Here's how the part is built. I have some questions about the finished solid (model axes, mm). Face numbers are marked on the shaded views. A direction names the side the tool comes from. Coordinates: 2 decimals unless noted, no trailing zeros. Order: outer loops, then holes, each group sorted by start corner. A loop starts at its lowest first (then second) coordinate and runs counter-clockwise, first axis right, second up. Notation, with made-up numbers: (64.5, 10) - (114.5, 10) arc R14 cw to (114.5, 25) - close; hole circle Ø10 at (4, -23). An arc over 180 degrees is marked (long way). Answer in a Markdown table with one row per item. Add a question column.
Item 1: I want a section at C-C (z = 4). Please give me the cut outline in (x, y) (3 decimals), plus the area to 3 significant figures.
Item 2: I want a section at D-D (z = 16). Please give me the cut outline in (x, y).
Item 3: On a 3-axis mill with a long thin cutter (end or side, diameter ignored), from which of +Z, -Z, +X, -X, +Y, -Y can I reach the whole of each face in a straight line? I mean the marked faces 4, 5, 6, 7 and 8. Say none if no direction works.
Item 4: If I drill on line 1 along Y through (x, z) = (54, 6); line 2 along Y through (x, z) = (22.5, 32); line 3 along Z through (x, y) = (24.5, -14.5), over which ranges is the centre line in solid material (lowest first)? Write a range as from..to.
Item 5: Will these pins go through, and if not, where does the flat tip stop? pin 1 Ø1 at (x, y) = (53, -6.5) entering from +Z; pin 2 Ø19 at (x, z) = (19, 27) entering from -Y; pin 3 Ø10 at (x, z) = (12.7, 31.75) entering from -Y; pin 4 Ø10 at (y, z) = (-7, 34.5) entering from +X.
Item 6: I want a section at A-A (y = -3). Please give me the cut outline in (x, z).
Item 7: Thinking about a two-plate mould opening in X: for the marked faces 1, 2 and 3, which applies, +X half, -X half, draft (parallel to the pull), parting line (faces both ways), or undercut?
Item 8: I want a section at B-B (z = 30). Please give me the cut outline in (x, y).
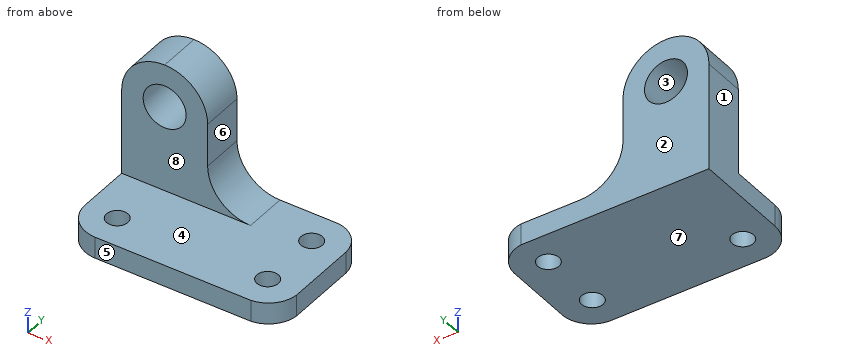
```python
from build123d import *

# Parameters (mm, degrees)
F0_W      = 63.5
F0_H      = 44.45
F1_DEPTH  = 38.1
F2_W      = 25.4
F2_H      = 38.1
F3_DEPTH  = 38.101
F5_W      = 25.4
F5_H      = 38.1
F6_DEPTH  = 38.101
F4_W      = 12.7
F4_H      = 25.4
F7_DEPTH  = 38.101
F8_R      = 6.35
F9_DEPTH  = 12.701
F10_R     = 3.175
F11_DEPTH = 6.351


# Not quite as in the source:
# - a feature names something its author has since deleted; it is built from what else it names


with BuildPart() as f1:
    # F0 (on Front) → F1 (new body)
    with BuildSketch(Plane.XZ):
        with Locations((31.75, 22.225)):
            Rectangle(F0_W, F0_H)
    extrude(amount=F1_DEPTH)

    # F2 (on face) → F3 (cut, through all)
    with BuildSketch(Plane.XZ.offset(38.1)):
        with Locations((50.8, 25.4)):
            Rectangle(F2_W, F2_H)
    extrude(amount=-F3_DEPTH, mode=Mode.SUBTRACT)

    # F5 (on face) → F6 (cut, through all)
    with BuildSketch(Plane.YZ.offset(38.1)):
        with Locations((-25.4, 25.4)):
            Rectangle(F5_W, F5_H)
    extrude(amount=-F6_DEPTH, mode=Mode.SUBTRACT)

    # F4 (on face) → F7 (cut, through all)
    with BuildSketch(Plane.XZ.offset(38.1)):
        with Locations((31.75, 31.75)):
            Rectangle(F4_W, F4_H)
        with BuildLine():
            Line((38.1, 19.05), (25.4, 19.05))
            ThreePointArc((25.4, 19.05), (29.1197438789, 10.0697438789), (38.1, 6.35))
            Line((38.1, 6.35), (38.1, 19.05))
        make_face()
    extrude(amount=-F7_DEPTH, mode=Mode.SUBTRACT)

    # F8 (on face) → F9 (cut, through all)
    with BuildSketch(Plane.XZ.offset(12.7)):
        with Locations((12.7, 31.75)):
            Circle(F8_R)
        with BuildLine():
            ThreePointArc((12.6999999213, 44.45), (21.6802560932, 40.7302561489), (25.4, 31.75))
            Line((25.4, 31.75), (25.4, 44.45))
            Line((25.4, 44.45), (12.6999999213, 44.45))
        make_face()
        with BuildLine():
            ThreePointArc((0, 31.75), (3.7197438511, 40.7302560932), (12.6999999213, 44.45))
            Line((12.6999999213, 44.45), (0, 44.45))
            Line((0, 44.45), (0, 31.75))
        make_face()
    extrude(amount=-F9_DEPTH, mode=Mode.SUBTRACT)

    # F10 (on face) → F11 (cut, through all)
    with BuildSketch(Plane.XY.offset(6.35)):
        with BuildLine():
            Line((63.5, 0), (55.5319362459, 0))
            ThreePointArc((55.5319362459, 0), (61.0732443905, -2.8419244619), (63.5, -8.5772089198))
            Line((63.5, -8.5772089198), (63.5, 0))
        make_face()
        with BuildLine():
            ThreePointArc((63.5, -30.1359133542), (60.963360935, -35.563360935), (55.5359133542, -38.1))
            Line((55.5359133542, -38.1), (63.5, -38.1))
            Line((63.5, -38.1), (63.5, -30.1359133542))
        make_face()
        with BuildLine():
            ThreePointArc((9.525, -38.1), (2.8223237752, -35.2776762248), (0, -28.575))
            Line((0, -28.575), (0, -38.1))
            Line((0, -38.1), (9.525, -38.1))
        make_face()
        with Locations((9.525, -28.575)):
            Circle(F10_R)
        with Locations((53.975, -28.575)):
            Circle(F10_R)
        with Locations((53.975, -9.525)):
            Circle(F10_R)
    extrude(amount=-F11_DEPTH, mode=Mode.SUBTRACT)


solid = f1.part
```
Values follow:
| question | item | result |
|---|---|---|
| 1 | outline | (0, -28.575) arc R9.638 ccw to (9.525, -38.1) - (55.536, -38.1) arc R8.779 ccw to (63.5, -30.136) - (63.5, -8.577) arc R9.123 ccw to (55.532, 0) - (0, 0) - close; hole circle Ø6.35 at (9.525, -28.575); hole circle Ø6.35 at (53.975, -28.575); hole circle Ø6.35 at (53.975, -9.525) |
| 1 | area | 2,270 mm^2 |
| 2 | outline | (0, -12.7) - (25.77, -12.7) - (25.77, 0) - (0, 0) - close |
| 3 | face 4 | +Z, +X, -Y |
| 3 | face 5 | +Z, -Z, +X, -X, -Y |
| 3 | face 6 | +Z, +X, +Y, -Y |
| 3 | face 7 | -Z, +X, -X, +Y, -Y |
| 3 | face 8 | +Z, +X, -X, -Y |
| 4 | line 1 | y = -38.1..-31.75, -25.4..-12.7, -6.35..0 |
| 4 | line 2 | y = -12.7..0 |
| 4 | line 3 | z = 0..6.35 |
| 5 | pin 1 | stops at z = 6.35 |
| 5 | pin 2 | stops at y = -12.7 |
| 5 | pin 3 | passes through |
| 5 | pin 4 | stops at x = 25.4 |
| 6 | outline | (0, 0) - (61.22, 0) - (61.22, 6.35) - (38.1, 6.35) arc R12.7 cw to (25.4, 19.05) - (25.4, 31.75) arc R12.7 ccw to (0, 31.75) - close; hole circle Ø12.7 at (12.7, 31.75) |
| 7 | face 1 | -X half |
| 7 | face 2 | draft |
| 7 | face 3 | undercut |
| 8 | outline | (0, -12.7) - (6.6, -12.7) - (6.6, 0) - (0, 0) - close; (18.8, -12.7) - (25.4, -12.7) - (25.4, 0) - (18.8, 0) - close |
